Geometry: final body of the model. Coordinates: model frame, mm. Face numbers are marked on the shaded views. Give positions to 0.01 mm unless a question says otherwise; leave off trailing zeros. Write each loop counter-clockwise with the first axis right and the second up, starting at its lowest first coordinate (ties: lowest second). Pieces come first, ordered by that corner, then holes. Notation, with made-up numbers: M -21.75,45 L 6.25,45 A17 cw 6.25,50 Z; hole C 24,-10.5 d1. An arc over 180 degrees is marked long. Use a Markdown table: item, result. Add a question column.
1) Pin query (flat end, axial travel): pin 1 (4 mm diameter, centred on y = -1, z = 12, fed in from +X); pin 2 (10 mm diameter, centred on y = 3.5, z = -5.5, fed in from +X). Return the tip coordinate at first contact, or that it passes through.
2) Draft query along Z for the marked faces 1, 2 and 3. Return one class per face: +Z half, -Z half, draft (parallel to the pull), parting line (faces both ways), or undercut.
3) Section C-C on x = 1.5. Return the cut outline in (y, z) (3 decimals), then the cut area to 3 significant figures.
4) Section D-D on y = 19.05. Return the cut outline in (x, z) (1 decimal), then the cut area to 3 significant figures.
5) Line query: line 1 (Z direction, x = -3, y = 19.05) (3 decimals); line 2 (Z direction, x = 3.1, y = 0); line 3 (Y direction, x = -4.25, z = 19.5). Output: solid intervals per line, ascending.
6) Section A-A on z = 0. Return the cut outline in (x, y) (1 decimal), then the cut area to 3 significant figures.
```python
from build123d import *

# Parameters (mm, degrees)
F0_W     = 50.8
F0_H     = 50.8
F1_DEPTH = 4.7625
F2_R     = 10.16
F3_DEPTH = 9.525
F4_R     = 16.51
F5_DEPTH = 2.159
F6_R     = 3.175
F7_DEPTH = 9.525
F8_R     = 13.335
F9_DEPTH = 4.953


with BuildPart() as f1:
    # F0 (on Right) → F1 (new body, symmetric)
    with BuildSketch(Plane.YZ):
        Rectangle(F0_W, F0_H)
    extrude(amount=F1_DEPTH, both=True)

    # F2 (on face) → F3 (cut, through all)
    with BuildSketch(Plane.YZ.offset(4.7625)):
        Circle(F2_R)
    extrude(amount=-F3_DEPTH, mode=Mode.SUBTRACT)

    # F4 (on face) → F5 (cut)
    with BuildSketch(Plane.YZ.offset(4.7625)):
        Circle(F4_R)
    extrude(amount=-F5_DEPTH, mode=Mode.SUBTRACT)

    # F6 (on face) → F7 (cut, through all)
    with BuildSketch(Plane.YZ.offset(4.7625)):
        with Locations((-19.05, 19.05)):
            Circle(F6_R)
        with Locations((19.05, 19.05)):
            Circle(F6_R)
        with Locations((-19.05, -19.05)):
            Circle(F6_R)
        with Locations((19.05, -19.05)):
            Circle(F6_R)
    extrude(amount=-F7_DEPTH, mode=Mode.SUBTRACT)

    # F8 (on face) → F9 (cut)
    with BuildSketch(Plane.YZ.offset(4.7625)):
        Circle(F8_R)
    extrude(amount=-F9_DEPTH, mode=Mode.SUBTRACT)


solid = f1.part
```
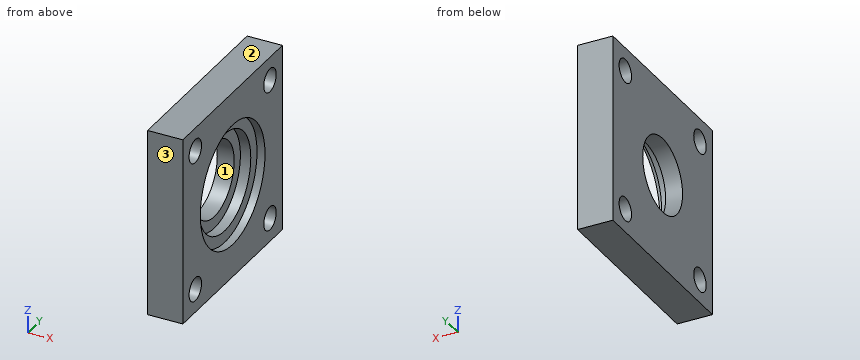
Found:
| question | item | result |
|---|---|---|
| 1 | pin 1 | x = 2.6 |
| 1 | pin 2 | x = -0.19 |
| 2 | face 1 | undercut |
| 2 | face 2 | +Z half |
| 2 | face 3 | draft |
| 3 | outline | M -25.4,-25.4 L 25.4,-25.4 L 25.4,25.4 L -25.4,25.4 Z; hole C -19.05,-19.05 d6.35; hole C -19.05,19.05 d6.35; hole C 0,0 d26.67; hole C 19.05,-19.05 d6.35; hole C 19.05,19.05 d6.35 |
| 3 | area | 1,900 mm² |
| 4 | outline | M -4.8,-25.4 L 4.8,-25.4 L 4.8,-22.2 L -4.8,-22.2 Z; M -4.8,-15.9 L 4.8,-15.9 L 4.8,15.9 L -4.8,15.9 Z; M -4.8,22.2 L 4.8,22.2 L 4.8,25.4 L -4.8,25.4 Z |
| 4 | area | 363 mm² |
| 5 | line 1 | -25.4 to -22.225, -15.875 to 15.875, 22.225 to 25.4 |
| 5 | line 2 | -25.4 to -16.51, 16.51 to 25.4 |
| 5 | line 3 | -25.4 to -22.19, -15.91 to 15.91, 22.19 to 25.4 |
| 6 | outline | M -4.8,-25.4 L 4.8,-25.4 L 4.8,-16.5 L 2.6,-16.5 L 2.6,-13.3 L -0.2,-13.3 L -0.2,-10.2 L -4.8,-10.2 Z; M -4.8,10.2 L -0.2,10.2 L -0.2,13.3 L 2.6,13.3 L 2.6,16.5 L 4.8,16.5 L 4.8,25.4 L -4.8,25.4 Z |
| 6 | area | 245 mm² |
